```python
from build123d import *

# Parameters (mm, degrees)
ESQUISSE1_W             = 85
ESQUISSE1_H             = 56
BOSS_EXTRU_1_DEPTH      = 2
ESQUISSE2_W             = 20
ESQUISSE2_H             = 15
ESQUISSE2_W_2           = 15
ESQUISSE2_H_2           = 13
BOSS_EXTRU_2_DEPTH      = 15
ESQUISSE3_R             = 1.5
ENL_V_MAT_EXTRU_1_DEPTH = 15
ESQUISSE5_R             = 2.5
ENL_V_MAT_EXTRU_2_DEPTH = 0.5
ESQUISSE6_W             = 50
ESQUISSE6_H             = 4
BOSS_EXTRU_3_DEPTH      = 9


with BuildPart() as part:
    # Esquisse1 → Boss.-Extru.1 (new body)
    with BuildSketch(Plane(origin=(0, 0, 0), x_dir=(0, 0, -1), z_dir=(1, 0, 0))):
        Rectangle(ESQUISSE1_W, ESQUISSE1_H)
    extrude(amount=BOSS_EXTRU_1_DEPTH)

    # Esquisse2 → Boss.-Extru.2 (add)
    with BuildSketch(Plane.ZY):
        with Locations((32.5, -16.5)):
            Rectangle(ESQUISSE2_W, ESQUISSE2_H)
        with Locations((35, 1.5)):
            Rectangle(ESQUISSE2_W_2, ESQUISSE2_H_2)
        with Locations((35, 18.5)):
            Rectangle(ESQUISSE2_W_2, ESQUISSE2_H_2)
    extrude(amount=BOSS_EXTRU_2_DEPTH)

    # Esquisse3 → Enlèv. mat.-Extru.1 (cut)
    with BuildSketch(Plane.ZY):
        with Locations((-38.5, 24.5)):
            Circle(ESQUISSE3_R)
        with Locations((19.5, 24.5)):
            Circle(ESQUISSE3_R)
        with Locations((-38.5, -24.5)):
            Circle(ESQUISSE3_R)
        with Locations((19.5, -24.5)):
            Circle(ESQUISSE3_R)
    extrude(amount=-ENL_V_MAT_EXTRU_1_DEPTH, mode=Mode.SUBTRACT)

    # Esquisse5 → Enlèv. mat.-Extru.2 (cut)
    with BuildSketch(Plane.ZY):
        with Locations((19.5, 24.5)):
            Circle(ESQUISSE5_R)
        with Locations((-38.5, 24.5)):
            Circle(ESQUISSE5_R)
        with Locations(Location((-38.5, -24.5, 0), (0, 0, 180))):
            Circle(ESQUISSE5_R)
        with Locations(Location((19.5, -24.5, 0), (0, 0, 180))):
            Circle(ESQUISSE5_R)
    extrude(amount=-ENL_V_MAT_EXTRU_2_DEPTH, mode=Mode.SUBTRACT)

    # Esquisse6 → Boss.-Extru.3 (add)
    with BuildSketch(Plane.ZY):
        with Locations((-9, 24)):
            Rectangle(ESQUISSE6_W, ESQUISSE6_H)
    extrude(amount=BOSS_EXTRU_3_DEPTH)


solid = part.part
```
The listing builds one solid part. Answer for the finished solid, in the listing's coordinates (mm). A direction names the side the tool comes from. Give positions to 0.01 mm unless a question says otherwise; leave off trailing zeros. Order: outer loops, then holes, each group sorted by start corner. A loop starts at its lowest first (then second) coordinate and runs counter-clockwise, first axis right, second up.
Item 1: The part is cut by section C-C, the plane x = -13.5. Give the vertices of the cut face in (y, z), and give its area (3 significant figures).
From the geometry:
outline: (-24, 22.5) - (-9, 22.5) - (-9, 42.5) - (-24, 42.5) - close; (-5, 27.5) - (8, 27.5) - (8, 42.5) - (-5, 42.5) - close; (12, 27.5) - (25, 27.5) - (25, 42.5) - (12, 42.5) - close
area: 690 mm2
Item 2: The part is cut by section B-B, the plane z = 19.5. Give the vertices of the cut face in (x, y), and give its area (3 significant figures).
From the geometry:
outline: (0, -28) - (2, -28) - (2, -26) - (0.5, -26) - (0.5, -27) - (0, -27) - close; (0, -22) - (0.5, -22) - (0.5, -23) - (2, -23) - (2, 23) - (0.5, 23) - (0.5, 22) - (0, 22) - close; (0, 27) - (0.5, 27) - (0.5, 26) - (2, 26) - (2, 28) - (0, 28) - close
area: 98.0 mm2
Item 3: The part is cut by section A-A, the plane x = -6.75. Give the vertices of the cut face in (y, z), and give its area (3 significant figures).
From the geometry:
outline: (-24, 22.5) - (-9, 22.5) - (-9, 42.5) - (-24, 42.5) - close; (-5, 27.5) - (8, 27.5) - (8, 42.5) - (-5, 42.5) - close; (12, 27.5) - (25, 27.5) - (25, 42.5) - (12, 42.5) - close; (22, -34) - (26, -34) - (26, 16) - (22, 16) - close
area: 890 mm2
Item 4: The part is cut by section D-D, the plane y = -18.5. Give the vertices of the cut face in (x, z).
From the geometry:
outline: (-15, 22.5) - (0, 22.5) - (0, -42.5) - (2, -42.5) - (2, 42.5) - (-15, 42.5) - close
Item 5: Which of the six approach directions +Z, -Z, +X, -X, +Y, -Y give full straight-line access (tool end or side, diameter ignored) to faces 1 (the face through (-9, 24, -9)), 2 (the face through (-7, 25, 35)), 3 (the face through (-7, -24, 32)), 4 (the face through (-7, -5, 35)), 5 (the face through (0.25, 26.61, -37.16))?
From the geometry:
face 1: -Z, -X, +Y, -Y
face 2: +Z, -X, +Y
face 3: +Z, -Z, -X, -Y
face 4: +Z, -Z, -X
face 5: -X
Item 6: Given pin 1 Ø4.5 at (y, z) = (24.5, 19.5) entering from -X; pin 2 Ø7.5 at (x, z) = (-5.5, 33.5) entering from -Y; pin 3 Ø4 at (y, z) = (24.5, -38.5) entering from +X; pin 4 Ø6 at (y, z) = (-24.5, 19.5) entering from -X, each flat-ended and moving along its own axis, determine where each tip first touches the part or whether it passes through.
From the geometry:
pin 1: stops at x = 0.5
pin 2: stops at y = -24
pin 3: stops at x = 2
pin 4: stops at x = 0
Item 7: For a pull along Z with two mould halves and no side action, classify faces 6 (the face through (0.25, -26.19, 21.34)), 7 (the face through (-7, 1, 27.5)), 8 (the face through (-7, -9, 32)) as pulls with the +Z half, pulls with the -Z half, needs draft (parallel to the pull), parting line crosses it, or undercut.
From the geometry:
face 6: undercut
face 7: pulls with the -Z half
face 8: needs draft
Item 8: Find the intervals of material crossed by probe 1 along Y at (x, z) = (0.35, -38.5); probe 2 along Y at (x, z) = (1.4, 19.5); probe 3 along Z at (x, y) = (0.3, -24.5), in increasing order.
From the geometry:
probe 1: y = -28 to -27, -22 to 22, 27 to 28
probe 2: y = -28 to -26, -23 to 23, 26 to 28
probe 3: z = -42.5 to -41, -36 to 17, 22 to 42.5
